Check sheet for the modelled part. Datum: model origin and axes. Units: mm. Give positions to 0.01 mm unless a question says otherwise; leave off trailing zeros. Loops run counter-clockwise (first coordinate to the right, second up) from the corner with the lowest first, then second, coordinate; pieces in that order, holes last. Notation, with made-up numbers: (11, -20) -> (49, -20) arc R22 ccw to (49, 11) -> close; hole circle Ø6 at (19, 57). An arc over 180 degrees is marked (long way). Answer as CSV lines item,"result". Start each with the question number.
(1) Material ranges on line 1 (Z direction, x = -82.5, y = 0.6); line 2 (X direction, y = 0.2, z = 213); line 3 (Z direction, x = -154, y = 0.55), recorded low to high. Write a range as from..to.
(2) Section check B-B on z = 278. Enter the section's corners in (x, y), plus the area to 3 significant figures.
(3) Release check for a two-part mould opening along Z. For faces 1 (the face through (-96, 0, 206)), 2 (the face through (-113.65, 0.79, 239.94)), 3 (the face through (-83.65, 0.79, 209.94)), 4 (the face through (-160.374, 0.789, 302.141)) record: pulls with the +Z half, pulls with the -Z half, needs draft (parallel to the pull), parting line crosses it, or undercut.
(4) Section check C-C on y = 1.1. State how many separate pieces and enclosed holes the cut face has, plus the area to 3 significant figures.
(5) Section check A-A on x = -107. Enter the section's corners in (y, z).
(6) Gauge pin test, flat ends, axial feed: pin 1 Ø3.5 at (x, z) = (-77.64, 226.89) entering from -Y; pin 2 Ø0.8 at (x, y) = (-93, 1) entering from -Z; pin 3 Ø0.5 at (y, z) = (1, 136.5) entering from +X. Record the tip position at first contact, or that the pin passes through.
from build123d import *

# Parameters (mm, degrees)
SKETCH1_R        = 2.2
SKETCH1_R_2      = 1.85915493
SKETCH1_R_3      = 2
SKETCH1_R_4      = 1.8
SKETCH1_R_5      = 1.673239437
SKETCH1_R_6      = 1.983111479
EXTRUSION1_DEPTH = 1.6
FILLET1_R        = 1
FILLET2_R        = 4
FILLET3_R        = 3
FILLET4_R        = 3
FILLET5_R        = 2
FILLET6_R        = 2
FILLET7_R        = 3
FILLET8_R        = 3
FILLET9_R        = 2
FILLET10_R       = 2
FILLET11_R       = 3


with BuildPart() as part:
    # Sketch1 → Extrusion1 (new body)
    with BuildSketch(Plane(origin=(0, 0, 0), x_dir=(-1, 0, 0), z_dir=(0, 1, 0))):
        Polygon((74.087520418, 321.088295015), (70.369210559, 327.285477572), (45.580478165, 327.285477572), (45.580478165, 312.412238135), (23.246043749, 290.934342561), (26.682507041, 287.360833055), (12.735407819, 253.538985229), (9.017097883, 253.538985229), (9.017097883, 226.891111382), (9.017097883, 200.243237534), (12.735407819, 200.243237534), (26.682507041, 166.421389708), (23.246043749, 162.847880202), (45.580478165, 141.369984628), (45.580478165, 126.496745191), (70.369210559, 126.496745191), (74.087520418, 132.693927748), (97.636816193, 132.693927748), (121.186111968, 132.693927748), (124.904421827, 126.496745191), (149.693154221, 126.496745191), (149.693154221, 141.369984628), (172.027588636, 162.847880202), (168.591125345, 166.421389708), (182.538224567, 200.243237534), (186.256534503, 200.243237534), (186.256534503, 226.891111382), (186.256534503, 253.538985229), (182.538224567, 253.538985229), (168.591125345, 287.360833055), (172.027588636, 290.934342561), (149.693154221, 312.412238135), (149.693154221, 327.285477572), (124.904421827, 327.285477572), (121.186111968, 321.088295015), (97.636816193, 321.088295015), align=None)
        with Locations((112.636816193, 211.891111382)):
            Circle(SKETCH1_R, mode=Mode.SUBTRACT)
        with Locations((49.266182018, 151.62213525)):
            Circle(SKETCH1_R_2, mode=Mode.SUBTRACT)
        with Locations((112.636816193, 241.891111382)):
            Circle(SKETCH1_R, mode=Mode.SUBTRACT)
        with Locations((82.636816193, 241.891111382)):
            Circle(SKETCH1_R, mode=Mode.SUBTRACT)
        with Locations((82.636816193, 211.891111382)):
            Circle(SKETCH1_R, mode=Mode.SUBTRACT)
        with Locations((117.636816193, 226.891111382)):
            Circle(SKETCH1_R_3, mode=Mode.SUBTRACT)
        with Locations((77.636816193, 226.891111382)):
            Circle(SKETCH1_R_3, mode=Mode.SUBTRACT)
        with Locations((97.636816193, 226.891111382)):
            Circle(SKETCH1_R_3, mode=Mode.SUBTRACT)
        with Locations((176.256534503, 218.641111382)):
            Circle(SKETCH1_R_4, mode=Mode.SUBTRACT)
        with Locations((176.256534503, 235.141111382)):
            Circle(SKETCH1_R_4, mode=Mode.SUBTRACT)
        with Locations((19.017097883, 218.641111382)):
            Circle(SKETCH1_R_4, mode=Mode.SUBTRACT)
        with Locations((19.017097883, 235.141111382)):
            Circle(SKETCH1_R_4, mode=Mode.SUBTRACT)
        with Locations((51.777661187, 316.130534525)):
            Circle(SKETCH1_R_2, mode=Mode.SUBTRACT)
        with Locations((49.266182018, 302.160087513)):
            Circle(SKETCH1_R_2, mode=Mode.SUBTRACT)
        with Locations((13.355125975, 240.524915841)):
            Circle(SKETCH1_R_5, mode=Mode.SUBTRACT)
        with Locations((143.495971199, 137.651688238)):
            Circle(SKETCH1_R_2, mode=Mode.SUBTRACT)
        with Locations((146.007450368, 151.62213525)):
            Circle(SKETCH1_R_2, mode=Mode.SUBTRACT)
        with Locations((143.495971199, 316.130534525)):
            Circle(SKETCH1_R_2, mode=Mode.SUBTRACT)
        with Locations((181.918506411, 240.524915841)):
            Circle(SKETCH1_R_5, mode=Mode.SUBTRACT)
        with Locations((146.007450368, 302.160087513)):
            Circle(SKETCH1_R_2, mode=Mode.SUBTRACT)
        with Locations((181.918506411, 213.257306923)):
            Circle(SKETCH1_R_5, mode=Mode.SUBTRACT)
        with Locations((13.355125975, 213.257306923)):
            Circle(SKETCH1_R_5, mode=Mode.SUBTRACT)
        with Locations((51.777661187, 137.651688238)):
            Circle(SKETCH1_R_2, mode=Mode.SUBTRACT)
        with Locations((67.636816193, 196.891111382)):
            Circle(SKETCH1_R_6, mode=Mode.SUBTRACT)
        with Locations((67.636816193, 256.891111382)):
            Circle(SKETCH1_R_6, mode=Mode.SUBTRACT)
        with Locations((42.888078851, 158.000238416)):
            Circle(SKETCH1_R_2, mode=Mode.SUBTRACT)
        with Locations((152.385553534, 295.781984347)):
            Circle(SKETCH1_R_2, mode=Mode.SUBTRACT)
        with Locations((42.888078851, 295.781984347)):
            Circle(SKETCH1_R_2, mode=Mode.SUBTRACT)
        with Locations((127.636816193, 256.891111382)):
            Circle(SKETCH1_R_6, mode=Mode.SUBTRACT)
        with Locations((152.385553534, 158.000238416)):
            Circle(SKETCH1_R_2, mode=Mode.SUBTRACT)
        with Locations((127.636816193, 196.891111382)):
            Circle(SKETCH1_R_6, mode=Mode.SUBTRACT)
    extrude(amount=EXTRUSION1_DEPTH)

    # Fillet1
    fillet1_edges = [part.edges().sort_by_distance(p)[0] for p in [
        (-121.186111968, 0.8, 321.088295015),
        (-121.186111968, 0.8, 132.693927748),
        (-74.087520418, 0.8, 132.693927748),
        (-74.087520418, 0.8, 321.088295015),
    ]]
    fillet(fillet1_edges, radius=FILLET1_R)

    # Fillet2
    fillet2_edges = [part.edges().sort_by_distance(p)[0] for p in [
        (-149.693154221, 0.8, 327.285477572),
        (-149.693154221, 0.8, 126.496745191),
        (-45.580478165, 0.8, 126.496745191),
        (-45.580478165, 0.8, 327.285477572),
    ]]
    fillet(fillet2_edges, radius=FILLET2_R)

    # Fillet3
    fillet3_edges = [part.edges().sort_by_distance(p)[0] for p in [
        (-149.693154221, 0.8, 312.412238135),
        (-149.693154221, 0.8, 141.369984628),
        (-45.580478165, 0.8, 141.369984628),
        (-45.580478165, 0.8, 312.412238135),
    ]]
    fillet(fillet3_edges, radius=FILLET3_R)

    # Fillet4
    fillet4_edges = [part.edges().sort_by_distance(p)[0] for p in [
        (-172.027588636, 0.8, 290.934342561),
    ]]
    fillet(fillet4_edges, radius=FILLET4_R)

    # Fillet5
    fillet5_edges = [part.edges().sort_by_distance(p)[0] for p in [
        (-168.591125345, 0.8, 287.360833055),
    ]]
    fillet(fillet5_edges, radius=FILLET5_R)

    # Fillet6
    fillet6_edges = [part.edges().sort_by_distance(p)[0] for p in [
        (-26.682507041, 0.8, 287.360833055),
    ]]
    fillet(fillet6_edges, radius=FILLET6_R)

    # Fillet7
    fillet7_edges = [part.edges().sort_by_distance(p)[0] for p in [
        (-23.246043749, 0.8, 290.934342561),
    ]]
    fillet(fillet7_edges, radius=FILLET7_R)

    # Fillet8
    fillet8_edges = [part.edges().sort_by_distance(p)[0] for p in [
        (-172.027588636, 0.8, 162.847880202),
        (-23.246043749, 0.8, 162.847880202),
    ]]
    fillet(fillet8_edges, radius=FILLET8_R)

    # Fillet9
    fillet9_edges = [part.edges().sort_by_distance(p)[0] for p in [
        (-168.591125345, 0.8, 166.421389708),
        (-26.682507041, 0.8, 166.421389708),
    ]]
    fillet(fillet9_edges, radius=FILLET9_R)

    # Fillet10
    fillet10_edges = [part.edges().sort_by_distance(p)[0] for p in [
        (-182.538224567, 0.8, 253.538985229),
        (-182.538224567, 0.8, 200.243237534),
        (-12.735407819, 0.8, 200.243237534),
        (-12.735407819, 0.8, 253.538985229),
    ]]
    fillet(fillet10_edges, radius=FILLET10_R)

    # Fillet11
    fillet11_edges = [part.edges().sort_by_distance(p)[0] for p in [
        (-186.256534503, 0.8, 200.243237534),
        (-186.256534503, 0.8, 253.538985229),
        (-9.017097883, 0.8, 253.538985229),
        (-9.017097883, 0.8, 200.243237534),
    ]]
    fillet(fillet11_edges, radius=FILLET11_R)


solid = part.part
Working result:
1,line 1,"z = 132.69..209.7, 214.09..239.7, 244.09..321.09"
1,line 2,"x = -186.26..-183.57, -180.27..-114.54, -110.74..-84.54, -80.74..-15.01, -11.7..-9.02"
1,line 3,"z = 145.51..157.08, 158.92..294.86, 296.7..308.27"
2,outline,"(-172.45, 0) -> (-22.82, 0) -> (-22.82, 1.6) -> (-172.45, 1.6) -> close"
2,area,"239 mm^2"
3,face 1,"needs draft"
3,face 2,"undercut"
3,face 3,"undercut"
3,face 4,"pulls with the +Z half"
4,separate pieces,"1"
4,enclosed holes,"31"
4,area,"28,500 mm^2"
5,outline,"(0, 132.69) -> (1.6, 132.69) -> (1.6, 321.09) -> (0, 321.09) -> close"
6,pin 1,"passes through"
6,pin 2,"stops at z = 132.69"
6,pin 3,"stops at x = -45.58"
